```python
from build123d import *

# Parameters (mm, degrees)
BOSS_EXTRUDE1_DEPTH = 3.175
SKETCH2_R           = 1.5
CUT_EXTRUDE1_DEPTH  = 154.964138984
SKETCH4_R           = 1.5
CUT_EXTRUDE2_DEPTH  = 154.964138984
SKETCH5_W           = 15
SKETCH5_H           = 30
SKETCH5_R           = 1.5
BOSS_EXTRUDE2_DEPTH = 3.175
SKETCH6_R           = 1.5
CUT_EXTRUDE3_DEPTH  = 159.599807878


with BuildPart() as part:
    # Sketch1 → Boss-Extrude1 (new body)
    with BuildSketch(Plane(origin=(0, 0, 0), x_dir=(1, 0, 0), z_dir=(0, 1, 0))):
        Polygon((110.595057034, -9.673003802), (95.595057034, -9.673003802), (95.595057034, -62.673003802), (118.095057034, -62.673003802), (118.095057034, -47.673003802), (110.595057034, -47.673003802), align=None)
        Polygon((95.595057034, 43.326996198), (95.595057034, -9.673003802), (110.595057034, -9.673003802), (110.595057034, 28.326996198), (118.095057034, 28.326996198), (118.095057034, 43.326996198), align=None)
        Polygon((140.595057034, 43.326996198), (118.095057034, 43.326996198), (118.095057034, 28.326996198), (125.595057034, 28.326996198), (125.595057034, -9.673003802), (140.595057034, -9.673003802), align=None)
        Polygon((118.095057034, -47.673003802), (118.095057034, -62.673003802), (140.595057034, -62.673003802), (140.595057034, -9.673003802), (125.595057034, -9.673003802), (125.595057034, -47.673003802), align=None)
    extrude(amount=BOSS_EXTRUDE1_DEPTH)

    # Sketch2 → Cut-Extrude1 (cut, through all)
    with BuildSketch(Plane.XZ):
        with Locations(Location((128.095812091, -40.826241141, 0), (0, 0, 270))):
            Circle(SKETCH2_R)
        with Locations(Location((138.094301977, -40.826241141, 0), (0, 0, 270))):
            Circle(SKETCH2_R)
        with Locations(Location((138.094301977, -30.827751255, 0), (0, 0, 270))):
            Circle(SKETCH2_R)
        with Locations(Location((128.095812091, -30.827751255, 0), (0, 0, 270))):
            Circle(SKETCH2_R)
        with Locations(Location((138.094301977, 60.172248745, 0), (0, 0, 90))):
            Circle(SKETCH2_R)
        with Locations(Location((138.094301977, 50.173758859, 0), (0, 0, 90))):
            Circle(SKETCH2_R)
        with Locations(Location((128.095812091, 50.173758859, 0), (0, 0, 90))):
            Circle(SKETCH2_R)
        with Locations(Location((128.095812091, 60.172248745, 0), (0, 0, 90))):
            Circle(SKETCH2_R)
        with Locations(Location((98.095812091, -40.826241141, 0), (0, 0, 90))):
            Circle(SKETCH2_R)
        with Locations(Location((98.095812091, -30.827751255, 0), (0, 0, 90))):
            Circle(SKETCH2_R)
        with Locations(Location((108.094301977, -30.827751255, 0), (0, 0, 90))):
            Circle(SKETCH2_R)
        with Locations(Location((108.094301977, -40.826241141, 0), (0, 0, 90))):
            Circle(SKETCH2_R)
        with Locations(Location((98.095812091, 50.173758859, 0), (0, 0, 270))):
            Circle(SKETCH2_R)
        with Locations(Location((98.095812091, 60.172248745, 0), (0, 0, 270))):
            Circle(SKETCH2_R)
        with Locations(Location((108.094301977, 60.172248745, 0), (0, 0, 270))):
            Circle(SKETCH2_R)
        with Locations(Location((108.094301977, 50.173758859, 0), (0, 0, 270))):
            Circle(SKETCH2_R)
    extrude(amount=-CUT_EXTRUDE1_DEPTH, mode=Mode.SUBTRACT)

    # Sketch4 → Cut-Extrude2 (cut, through all)
    with BuildSketch(Plane.XZ):
        with Locations(Location((133.095057034, 32.673003802, 0), (0, 0, 270))):
            Circle(SKETCH4_R)
        with Locations(Location((133.095057034, -13.549475249, 0), (0, 0, 270))):
            Circle(SKETCH4_R)
        with Locations(Location((103.095057034, -13.549475249, 0), (0, 0, 90))):
            Circle(SKETCH4_R)
        with Locations(Location((103.095057034, 32.673003802, 0), (0, 0, 90))):
            Circle(SKETCH4_R)
    extrude(amount=-CUT_EXTRUDE2_DEPTH, mode=Mode.SUBTRACT)

    # Sketch5 → Boss-Extrude2 (add)
    # profile 1 of 2: a face of its own
    with BuildSketch(Plane.XZ):
        with Locations((133.095057034, -58.326996198)):
            Rectangle(SKETCH5_W, SKETCH5_H)
        Polygon((133.095057034, -58.326996198), (133.117194018, -58.371270165), (133.095057034, -58.415806265), align=None, mode=Mode.SUBTRACT)
        with Locations(Location((133.095057034, -50.915806265, 0), (0, 0, 270))):
            Circle(SKETCH5_R, mode=Mode.SUBTRACT)
        with Locations(Location((133.095057034, -65.915806265, 0), (0, 0, 270))):
            Circle(SKETCH5_R, mode=Mode.SUBTRACT)
    # profile 2 of 2: a face of its own
    with BuildSketch(Plane.XZ):
        with Locations((103.095057034, -58.326996198)):
            Rectangle(SKETCH5_W, SKETCH5_H)
        with Locations(Location((103.095057034, -65.915806265, 0), (0, 0, 270))):
            Circle(SKETCH5_R, mode=Mode.SUBTRACT)
        with Locations(Location((103.095057034, -50.915806265, 0), (0, 0, 270))):
            Circle(SKETCH5_R, mode=Mode.SUBTRACT)
    extrude(amount=-BOSS_EXTRUDE2_DEPTH)

    # Sketch6 → Cut-Extrude3 (cut, through all)
    with BuildSketch(Plane(origin=(0, 3.175, 0), x_dir=(1, 0, 0), z_dir=(0, 1, 0))):
        with Locations(Location((118.095057034, -55.173003802, 0), (0, 0, 270))):
            Circle(SKETCH6_R)
        with Locations(Location((118.095057034, 35.826996198, 0), (0, 0, 90))):
            Circle(SKETCH6_R)
    extrude(amount=-CUT_EXTRUDE3_DEPTH, mode=Mode.SUBTRACT)


solid = part.part
```
Build history of the part. All positions in model axes, mm. A direction names the side the tool comes from. Round coordinates to 2 decimals unless told otherwise and drop trailing zeros. Loops run counter-clockwise (first coordinate to the right, second up) from the corner with the lowest first, then second, coordinate; pieces in that order, holes last.
Item 1: Pin check, flat tips, straight feed: P1, Ø3.5, axis at x = 128.1, z = 50.17, coming from the -Y side; P2, Ø1.8, axis at x = 98.1, z = 50.17, coming from the +Y side; P3, Ø1, axis at x = 117, y = 1.5, coming from the -Z side. Stop position of each tip, or through.
Item 2: Two-plate mould, pull along X, no slides. Class faces 1 (the face through (96.83, 1.57, -30.02)), 2 (the face through (95.595, 2, -6)), 3 (the face through (103, 2, -73.327)): released by +X, released by -X, zero draft, split by the parting line, or undercut.
Item 3: Saw through at B-B (z = 28.5). List the corners of the cut face in (x, y) (3 decimals).
Item 4: Saw through at A-A (x = 122.5). List the corners of the cut face in (y, z) (3 decimals).
Item 5: Drill centre lines: line 1 along X through (y, z) = (2.65, -66); line 2 along X through (y, z) = (2.95, 25); line 3 along Z through (x, y) = (122.5, 0.9). Where is each one in solid material? Low to high.
Item 6: Which spindle directions (+Z, -Z, +X, -X, +Y, -Y) get a long thin tool onto all of the face, cutting with end or side? Do faces 4 (the face through (118, 2, -43.327)), 5 (the face through (119.01, 1.61, -34.64)). Say none if no direction does.
Worked answers:
1. P1: stops at y = 0
1. P2: passes through
1. P3: stops at z = -43.33
2. face 1: undercut
2. face 2: released by -X
2. face 3: zero draft
3. outline: (95.595, 0) - (110.595, 0) - (110.595, 3.175) - (95.595, 3.175) - close; (125.595, 0) - (140.595, 0) - (140.595, 3.175) - (125.595, 3.175) - close
4. outline: (0, -43.327) - (3.175, -43.327) - (3.175, -28.327) - (0, -28.327) - close; (0, 47.673) - (3.175, 47.673) - (3.175, 62.673) - (0, 62.673) - close
5. line 1: x = 95.6 to 101.6, 104.59 to 110.6, 125.6 to 131.6, 134.59 to 140.6
5. line 2: x = 95.6 to 110.6, 125.6 to 140.6
5. line 3: z = -43.33 to -28.33, 47.67 to 62.67
6. face 4: -Z, +Y, -Y
6. face 5: +Y, -Y
